Verification items for the finished model (mm, model axes). A direction names the side the tool comes from. Coordinates: 2 decimals unless noted, no trailing zeros. Write each loop counter-clockwise with the first axis right and the second up, starting at its lowest first coordinate (ties: lowest second). Pieces come first, ordered by that corner, then holes.
```python
from build123d import *

# Parameters (mm, degrees)
BOSS_EXTRUDE1_DEPTH = 135
SKETCH6_R           = 1.6
BOSS_EXTRUDE2_DEPTH = 2
FILLET3_R           = 5
FILLET4_R           = 2.5


with BuildPart() as part:
    # Sketch4 → Boss-Extrude1 (new body)
    with BuildSketch(Plane(origin=(0, 0, 0), x_dir=(1, 0, 0), z_dir=(0, 1, 0))):
        Polygon((-7.5, -7.5), (7.5, -7.5), (7.5, -6), (0, -6), (0, -3), (7.5, -3), (7.5, -1.5), (-1.5, -1.5), (-1.5, 7.5), (-3, 7.5), (-3, 0), (-6, 0), (-6, 7.5), (-7.5, 7.5), align=None)
    extrude(amount=BOSS_EXTRUDE1_DEPTH)

    # Sketch6 → Boss-Extrude2 (add)
    with BuildSketch(Plane.XZ):
        Polygon((7.5, 7.5), (-7.5, 7.5), (-7.5, -7.5), (-6, -7.5), (-6, 0), (-3, 0), (-3, -7.5), (-1.5, -7.5), (7.5, -7.5), (7.5, 1.5), (7.5, 3), (0, 3), (0, 6), (7.5, 6), align=None)
        with Locations((3, -3)):
            Circle(SKETCH6_R, mode=Mode.SUBTRACT)
    extrude(amount=BOSS_EXTRUDE2_DEPTH)

    # Fillet3
    fillet3_edges = [part.edges().sort_by_distance(p)[0] for p in [
        (-7.5, 66.5, 7.5),
    ]]
    fillet(fillet3_edges, radius=FILLET3_R)

    # Fillet4
    fillet4_edges = [part.edges().sort_by_distance(p)[0] for p in [
        (-1.5, 67.5, 1.5),
    ]]
    fillet(fillet4_edges, radius=FILLET4_R)


solid = part.part
```
1. Gauge pin test, flat ends, axial feed: P1, Ø2, axis at y = 68.5, z = -5, coming from the +X side; P2, Ø1.5, axis at x = -4, y = 86.5, coming from the +Z side; P3, Ø0.9, axis at x = -5, y = 88, coming from the -Z side. Record the tip position at first contact, or that the pin passes through.
2. Material ranges on L1, parallel to Z at x = 3, y = -0.45; L2, parallel to X at y = 37.5, z = -1.5; L3, parallel to Z at x = 3.75, y = 57.5, recorded low to high.
3. Draft check along Z on faces 5 (the flat face through (0, 67, 4)), 6 (the flat face through (4, 67, 3)), 7 (the cylindrical face through (-0.748, 68.445, 0.787)), 8 (the flat face through (3, 67, 7.5)). Enter one of: pulls with the +Z half, pulls with the -Z half, needs draft (parallel to the pull), parting line crosses it, or undercut.
4. Sectioned sample at B-B, the plane x = 3. Record the boundary of the cut face in (y, z), and give its area (3 significant figures).
5. Sectioned sample at D-D, the plane x = -4.25. Record the boundary of the cut face in (y, z), and give its area (3 significant figures).
6. Sectioned sample at A-A, the plane z = -3. Record the boundary of the cut face in (x, y), and give its area (3 significant figures).
7. Tool access check on faces 1 (the flat face through (4, 67, 6)), 2 (the flat face through (-6, 67, -4)), 3 (the flat face through (4, 67, 1.5)), 4 (the flat face through (-7.5, 67, -2)). Record the directions out of +Z, -Z, +X, -X, +Y, -Y that give a thin tool (end or side, any length) a straight path to the whole face; none if there is none.
8. Sectioned sample at C-C, the plane y = 43. Record the boundary of the cut face in (x, z), and give its area (3 significant figures).
Outcome:
1. P1: stops at x = -1.5
1. P2: stops at z = 7.44
1. P3: stops at z = 0
2. L1: z = -7.5 to -4.6, -1.4 to 3, 6 to 7.5
2. L2: x = -7.5 to -6, -3 to -1.5
2. L3: z = 1.5 to 3, 6 to 7.5
3. face 5: undercut
3. face 6: undercut
3. face 7: pulls with the -Z half
3. face 8: pulls with the +Z half
4. outline: (-2, -7.5) - (0, -7.5) - (0, -4.6) - (-2, -4.6) - close; (-2, -1.4) - (0, -1.4) - (0, 1.5) - (135, 1.5) - (135, 3) - (-2, 3) - close; (-2, 6) - (135, 6) - (135, 7.5) - (-2, 7.5) - close
4. area: 423 mm2
5. outline: (-2, 0) - (135, 0) - (135, 7.18) - (-2, 7.18) - close
5. area: 984 mm2
6. outline: (-7.5, -2) - (-6, -2) - (-6, 135) - (-7.5, 135) - close; (-3, -2) - (1.4, -2) - (1.4, 0) - (-1.5, 0) - (-1.5, 135) - (-3, 135) - close; (4.6, -2) - (7.5, -2) - (7.5, 0) - (4.6, 0) - close
6. area: 423 mm2
7. face 1: +X, +Y, -Y
7. face 2: -Z, +Y, -Y
7. face 3: -Z, +X, +Y
7. face 4: +Z, -Z, -X, +Y, -Y
8. outline: (-7.5, -7.5) - (-6, -7.5) - (-6, 0) - (-3, 0) - (-3, -7.5) - (-1.5, -7.5) - (-1.5, -1) arc R2.5 cw to (1, 1.5) - (7.5, 1.5) - (7.5, 3) - (0, 3) - (0, 6) - (7.5, 6) - (7.5, 7.5) - (-2.5, 7.5) arc R5 ccw to (-7.5, 2.5) - close
8. area: 95.0 mm2
